Could you check a few things on this drawing? It's one solid part, dimensions in mm from its lowest x, y, z. Coordinates: 2 decimals unless noted, no trailing zeros. Loops run counter-clockwise (first coordinate to the right, second up) from the corner with the lowest first, then second, coordinate; pieces in that order, holes last. Notation, with made-up numbers: M 52,-27.75 L 97,-27.75 A19 cw 97,7.25 Z; hole C 7.25,3 d2. An arc over 180 degrees is marked long. Answer as a JSON object with one key per item and string values. Group by question number.
Item 1: Suppose I cut it at B-B (x = 14.75). Write out the boundary of the cut face in (y, z).
Item 2: I'm going to push flat-ended pins straight in: pin 1 Ø0.6 at (y, z) = (4.5, 2.5) entering from -X; pin 2 Ø0.6 at (y, z) = (19.5, 3.5) entering from +X; pin 3 Ø5 at (x, y) = (10, 18.5) entering from +Z. Where does each tip first touch, or does it pass through?
Item 3: Suppose I cut it at A-A (z = 2.8). Write out the boundary of the cut face in (x, y), then the cut area to 3 significant figures.
Item 4: If I drill on line 1 (X direction, y = 31, z = 3.45); line 2 (X direction, y = 18, z = 3.4); line 3 (Y direction, x = 2.5, z = 2.1), over which ranges is the centre line in solid material (lowest first)?
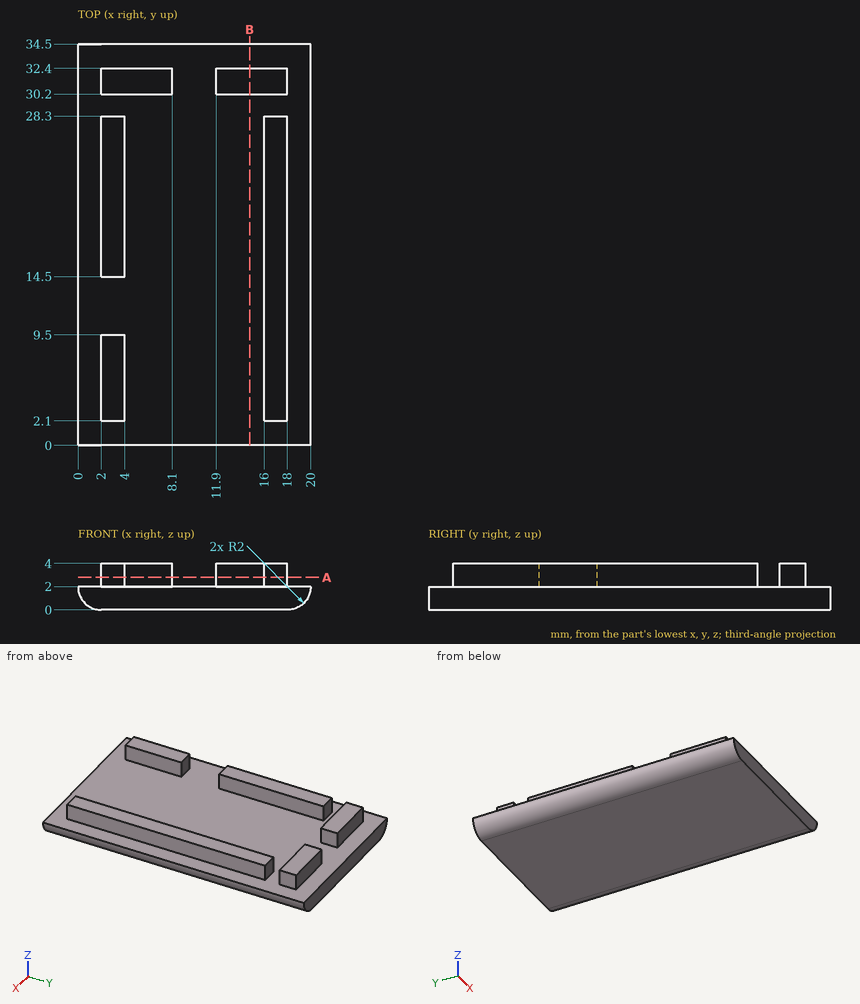
From the geometry:
{
 "1": {"outline": "M 0,0 L 34.5,0 L 34.5,2 L 32.4,2 L 32.4,4 L 30.2,4 L 30.2,2 L 0,2 Z"},
 "2": {"pin 1": "x = 2", "pin 2": "x = 18", "pin 3": "z = 2"},
 "3": {"outline": "M 2,2.1 L 4,2.1 L 4,9.5 L 2,9.5 Z; M 2,14.5 L 4,14.5 L 4,28.3 L 2,28.3 Z; M 2,30.2 L 8.1,30.2 L 8.1,32.4 L 2,32.4 Z; M 11.9,30.2 L 18,30.2 L 18,32.4 L 11.9,32.4 Z; M 16,2.1 L 18,2.1 L 18,28.3 L 16,28.3 Z", "area": "122 mm2"},
 "4": {"line 1": "2 to 8.1, 11.9 to 18", "line 2": "2 to 4, 16 to 18", "line 3": "2.1 to 9.5, 14.5 to 28.3, 30.2 to 32.4"}
}
